The model under review builds one solid part; all positions refer to its coordinate system, in mm. A direction names the side the tool comes from. Round coordinates to 2 decimals unless told otherwise and drop trailing zeros. Order: outer loops, then holes, each group sorted by start corner. A loop starts at its lowest first (then second) coordinate and runs counter-clockwise, first axis right, second up. Notation, with made-up numbers: (86, -28.75) -> (96, -28.75) arc R25 cw to (96, -4.75) -> close; hole circle Ø8 at (82, 40). An arc over 180 degrees is marked (long way). Use a Markdown table: item, result. Add a question column.
```python
from build123d import *

# Parameters (mm, degrees)
F0_R     = 12.5
F1_DEPTH = 1
F2_R     = 0.5
F3_DEPTH = 3
F4_R     = 3.5
F4_R_2   = 1.55
F5_DEPTH = 3.001


with BuildPart() as f1:
    # F0 (on Top) → F1 (new body)
    with BuildSketch(Plane.XY):
        Circle(F0_R)
    extrude(amount=F1_DEPTH)

    # F2 (on Top) → F3 (join)
    with BuildSketch(Plane.XY):
        with Locations((10.2, 3)):
            Circle(F2_R)
        with Locations((6.8, 6)):
            Circle(F2_R)
        with Locations((10.2, 0)):
            Circle(F2_R)
        with Locations((10.2, -3)):
            Circle(F2_R)
        with Locations((6.8, -6)):
            Circle(F2_R)
        with Locations((3.4, -6)):
            Circle(F2_R)
        with Locations((0, -6)):
            Circle(F2_R)
        with Locations((-3.4, -6)):
            Circle(F2_R)
        with Locations((-6.8, -6)):
            Circle(F2_R)
        with Locations((-10.2, -3)):
            Circle(F2_R)
        with Locations((-10.2, 0)):
            Circle(F2_R)
        with Locations((-10.2, 3)):
            Circle(F2_R)
        with Locations((-6.8, 6)):
            Circle(F2_R)
        with Locations((-3.4, 6)):
            Circle(F2_R)
        with Locations((0, 6)):
            Circle(F2_R)
        with Locations((3.4, 6)):
            Circle(F2_R)
        with Locations((-6.8, -3)):
            Circle(F2_R)
        with Locations((-6.8, 3)):
            Circle(F2_R)
        with Locations((-3.4, -3)):
            Circle(F2_R)
        with Locations((-3.4, 3)):
            Circle(F2_R)
        with Locations((6.8, -3)):
            Circle(F2_R)
        with Locations((3.4, -3)):
            Circle(F2_R)
        with Locations((6.8, 3)):
            Circle(F2_R)
        with Locations((3.4, 3)):
            Circle(F2_R)
        with Locations((6.8, 9)):
            Circle(F2_R)
        with Locations((3.4, 9)):
            Circle(F2_R)
        with Locations((0, 9)):
            Circle(F2_R)
        with Locations((-3.4, 9)):
            Circle(F2_R)
        with Locations((-6.8, 9)):
            Circle(F2_R)
        with Locations((10.2, 6)):
            Circle(F2_R)
        with Locations((6.8, -9)):
            Circle(F2_R)
        with Locations((3.4, -9)):
            Circle(F2_R)
        with Locations((-10.2, 6)):
            Circle(F2_R)
        with Locations((10.2, -6)):
            Circle(F2_R)
        with Locations((-3.4, -9)):
            Circle(F2_R)
        with Locations((0, -9)):
            Circle(F2_R)
        with Locations((-6.8, -9)):
            Circle(F2_R)
        with Locations((-10.2, -6)):
            Circle(F2_R)
    extrude(amount=F3_DEPTH)

    # F4 (on Top) → F5 (cut, through all)
    with BuildSketch(Plane.XY):
        Circle(F4_R)
        with Locations((8.15, 0)):
            Circle(F4_R_2)
        with Locations((-8.15, 0)):
            Circle(F4_R_2)
    extrude(amount=F5_DEPTH, mode=Mode.SUBTRACT)


solid = f1.part
```
Q1. Add section D-D (x = 10.2). Write out the cut boundary in (y, z).
Q2. Add section B-B (x = 0). Write out the cut boundary in (y, z).
Q3. Add section C-C (z = 1.8). State how many separate pieces and enclosed holes the cut face has, then the cut area to 3 significant figures.
Q4. Machinability: for faces 1 (the flat face through (0, 9, 3)), 2 (the cylindrical face through (-7.3, -6, 2)), which of the approach directions +Z, -Z, +X, -X, +Y, -Y give a long, thin tool a straight path to every point of the face, cutting with its end or side? Answer none if there is none.
Q5. Wall thickness on line 1 (X direction, y = 1.25, z = 0.65); line 2 (Y direction, x = 0, z = 0.35); line 3 (Z direction, x = -2.5, y = -11): over which ranges is each line inside the solid? List them lowest first. Write a range as [from, to].
Q6. Insertion check: pin 1 (1.5 mm diameter, centred on x = 7.5, z = 2, fed in from -Y). The pin has a flat end and moves straight along its axis. Give the tip position at first contact, or say it passes through.
Q7. Mouldability with a two-part tool opening along Y and no side actions: class faces 3 (the cylindrical face through (7.277, -2.85, 1.986)), 4 (the cylindrical face through (11.923, 3.755, 0.493)), 5 (the flat face through (7, -6, 3)) as pulls with the +Y half, pulls with the -Y half, needs draft (parallel to the pull), parting line crosses it, or undercut.
Report:
| question | item | result |
|---|---|---|
| 1 | outline | (-7.23, 0) -> (7.23, 0) -> (7.23, 1) -> (6.5, 1) -> (6.5, 3) -> (5.5, 3) -> (5.5, 1) -> (3.5, 1) -> (3.5, 3) -> (2.5, 3) -> (2.5, 1) -> (0.5, 1) -> (0.5, 3) -> (-0.5, 3) -> (-0.5, 1) -> (-2.5, 1) -> (-2.5, 3) -> (-3.5, 3) -> (-3.5, 1) -> (-5.5, 1) -> (-5.5, 3) -> (-6.5, 3) -> (-6.5, 1) -> (-7.23, 1) -> close |
| 2 | outline | (-12.5, 0) -> (-3.5, 0) -> (-3.5, 1) -> (-5.5, 1) -> (-5.5, 3) -> (-6.5, 3) -> (-6.5, 1) -> (-8.5, 1) -> (-8.5, 3) -> (-9.5, 3) -> (-9.5, 1) -> (-12.5, 1) -> close; (3.5, 0) -> (12.5, 0) -> (12.5, 1) -> (9.5, 1) -> (9.5, 3) -> (8.5, 3) -> (8.5, 1) -> (6.5, 1) -> (6.5, 3) -> (5.5, 3) -> (5.5, 1) -> (3.5, 1) -> close |
| 3 | separate pieces | 38 |
| 3 | enclosed holes | 0 |
| 3 | area | 29.8 mm² |
| 4 | face 1 | +Z, +X, -X, +Y, -Y |
| 4 | face 2 | +Z |
| 5 | line 1 | x = [-12.44, -9.07], [-7.23, -3.27], [3.27, 7.23], [9.07, 12.44] |
| 5 | line 2 | y = [-12.5, -3.5], [3.5, 12.5] |
| 5 | line 3 | z = [0, 1] |
| 6 | pin 1 | stops at y = -9.5 |
| 7 | face 3 | undercut |
| 7 | face 4 | parting line crosses it |
| 7 | face 5 | needs draft |
